Work out the finished part from the listing and answer in its coordinate system (mm). A direction names the side the tool comes from. Round coordinates to 2 decimals unless told otherwise and drop trailing zeros. Order: outer loops, then holes, each group sorted by start corner. A loop starts at its lowest first (then second) coordinate and runs counter-clockwise, first axis right, second up. Notation, with made-up numbers: M 45.25,-34.75 L 88.25,-34.75 A18 cw 88.25,-16.75 Z; hole C 71.5,48 d5. An arc over 180 degrees is marked long. Return JSON: item names as keys, results as strings.
from build123d import *

# Parameters (mm, degrees)
SKETCH1_W           = 1200.15
SKETCH1_H           = 600.075
BOSS_EXTRUDE1_DEPTH = 34.925
SKETCH2_R           = 20.213000011
BOSS_EXTRUDE2_DEPTH = 685.8
SKETCH3_R           = 51.963000011
BOSS_EXTRUDE3_DEPTH = 1.5875


with BuildPart() as part:
    # Sketch1 → Boss-Extrude1 (new body)
    with BuildSketch(Plane(origin=(0, 0, 0), x_dir=(1, 0, 0), z_dir=(0, 1, 0))):
        Rectangle(SKETCH1_W, SKETCH1_H)
    extrude(amount=BOSS_EXTRUDE1_DEPTH)

    # Sketch2 → Boss-Extrude2 (add)
    with BuildSketch(Plane.XZ):
        with Locations((-539.75, 239.7125)):
            Circle(SKETCH2_R)
        with Locations((539.75, 239.7125)):
            Circle(SKETCH2_R)
        with Locations((-539.75, -239.7125)):
            Circle(SKETCH2_R)
        with Locations((539.75, -239.7125)):
            Circle(SKETCH2_R)
    extrude(amount=BOSS_EXTRUDE2_DEPTH)

    # Sketch3 → Boss-Extrude3 (add)
    with BuildSketch(Plane.XZ):
        with Locations((-539.75, 239.7125)):
            Circle(SKETCH3_R)
        with Locations((539.75, 239.7125)):
            Circle(SKETCH3_R)
        with Locations((539.75, -239.7125)):
            Circle(SKETCH3_R)
        with Locations((-539.75, -239.7125)):
            Circle(SKETCH3_R)
    extrude(amount=BOSS_EXTRUDE3_DEPTH)


solid = part.part
Item 1: Find section A-A (x = -539.75). Determine the outline of the cut face in (y, z) (1 decimal).
Output:
{"outline": "M -685.8,-259.9 L -1.6,-259.9 L -1.6,-291.7 L 0,-291.7 L 0,-300 L 34.9,-300 L 34.9,300 L 0,300 L 0,291.7 L -1.6,291.7 L -1.6,259.9 L -685.8,259.9 L -685.8,219.5 L -1.6,219.5 L -1.6,187.7 L 0,187.7 L 0,-187.7 L -1.6,-187.7 L -1.6,-219.5 L -685.8,-219.5 Z"}
Item 2: Find section C-C (y = -46). Determine the outline of the cut face in (x, z), plus the area to 3 significant figures.
Output:
{"outline": "C -539.75,-239.71 d40.43; C -539.75,239.71 d40.43; C 539.75,-239.71 d40.43; C 539.75,239.71 d40.43", "area": "5,130 mm^2"}
Item 3: The mould has two halves that part along X. Classify faces 3 (the flat face through (539, -1.588, -262)), 4 (the flat face through (-8, 17, -300.038)), 5 (the flat face through (-600.075, 17, 4)): pulls with the +X half, pulls with the -X half, needs draft (parallel to the pull), parting line crosses it, or undercut.
Output:
{"face 3": "undercut", "face 4": "needs draft", "face 5": "pulls with the -X half"}
Item 4: Consider line 1 along Y through (x, z) = (53.5, 35.5) (3 decimals); line 2 along X through (y, z) = (-298, -245.5). Determine where each line is inside the solid, lowest interval first. Write a range as [from, to].
Output:
{"line 1": "y = [0, 34.925]", "line 2": "x = [-559.12, -520.38], [520.38, 559.12]"}
Item 5: Find section D-D (x = 430.5). Determine the outline of the cut face in (y, z) (1 decimal), plus the area to 3 significant figures.
Output:
{"outline": "M 0,-300 L 34.9,-300 L 34.9,300 L 0,300 Z", "area": "21,000 mm^2"}
Item 6: Which of the six approach directions +Z, -Z, +X, -X, +Y, -Y give full straight-line access (tool end or side, diameter ignored) to faces 1 (the flat face through (-8, 17, 300.038)), 2 (the cylindrical face through (559.03, -338.9, -233.64))?
Output:
{"face 1": "+Z, +X, -X, +Y, -Y", "face 2": "-Y"}
Item 7: This flat-tipped pin is pushed along its axis until it touches: pin 1 (3 mm diameter, centred on x = -356, z = -102.5, fed in from -Y). Where does it stop, or does it pass through?
Output:
{"pin 1": "stops at y = 0"}
Item 8: Find section B-B (z = 3). Determine the outline of the cut face in (x, y) (3 decimals).
Output:
{"outline": "M -600.075,0 L 600.075,0 L 600.075,34.925 L -600.075,34.925 Z"}
